```python
from build123d import *

# Parameters (mm, degrees)
ESBO_O1_W                = 2
ESBO_O1_H                = 2
RESSALTO_EXTRUS_O1_DEPTH = 100
RESSALTO_EXTRUS_O2_DEPTH = 2
RESSALTO_EXTRUS_O3_DEPTH = 2
ESBO_O4_R                = 1.75
CORTE_EXTRUS_O1_DEPTH    = 2
ESBO_O5_R                = 1.75
CORTE_EXTRUS_O2_DEPTH    = 2


with BuildPart() as part:
    # Esboço1 → Ressalto-extrusão1 (new body)
    with BuildSketch(Plane(origin=(0, 0, 0), x_dir=(1, 0, 0), z_dir=(0, 1, 0))):
        with Locations((1, 1)):
            Rectangle(ESBO_O1_W, ESBO_O1_H)
    extrude(amount=RESSALTO_EXTRUS_O1_DEPTH)

    # Esboço2 → Ressalto-extrusão2 (add)
    with BuildSketch(Plane.XY):
        Polygon((2, 0), (100, 0), (2, 100), align=None)
    extrude(amount=-RESSALTO_EXTRUS_O2_DEPTH)

    # Esboço3 → Ressalto-extrusão3 (add)
    with BuildSketch(Plane.ZY):
        Polygon((-2, 0), (-2, 100), (-100, 0), align=None)
    extrude(amount=-RESSALTO_EXTRUS_O3_DEPTH)

    # Esboço4 → Corte-extrusão1 (cut)
    with BuildSketch(Plane.ZY):
        with Locations((-10, 15)):
            Circle(ESBO_O4_R)
        with Locations((-10, 30)):
            Circle(ESBO_O4_R)
        with Locations((-10, 85)):
            Circle(ESBO_O4_R)
        with Locations((-10, 70)):
            Circle(ESBO_O4_R)
        with Locations((-55, 15)):
            Circle(ESBO_O4_R)
        with Locations((-70, 15)):
            Circle(ESBO_O4_R)
    extrude(amount=-CORTE_EXTRUS_O1_DEPTH, mode=Mode.SUBTRACT)

    # Esboço5 → Corte-extrusão2 (cut)
    with BuildSketch(Plane.XY):
        with Locations((10, 15)):
            Circle(ESBO_O5_R)
        with Locations((10, 30)):
            Circle(ESBO_O5_R)
        with Locations((10, 85)):
            Circle(ESBO_O5_R)
        with Locations((10, 70)):
            Circle(ESBO_O5_R)
        with Locations((70, 15)):
            Circle(ESBO_O5_R)
        with Locations((55, 15)):
            Circle(ESBO_O5_R)
    extrude(amount=-CORTE_EXTRUS_O2_DEPTH, mode=Mode.SUBTRACT)


solid = part.part
```
Design review of the part built by this model. Coordinates are the model's own, in mm. A direction names the side the tool comes from. Give positions to 0.01 mm unless a question says otherwise; leave off trailing zeros. Order: outer loops, then holes, each group sorted by start corner. A loop starts at its lowest first (then second) coordinate and runs counter-clockwise, first axis right, second up. Notation, with made-up numbers: (-30, 43.5) - (14, 43.5) arc R35 cw to (14, 82.5) - close; hole circle Ø10 at (65.5, 88.25). An arc over 180 degrees is marked (long way). Use a Markdown table: item, result. Add a question column.
(1) Add section D-D on y = 30. Give the boundary of the cut face in (x, z).
(2) Mouldability with a two-part tool opening along Z and no side actions: class faces 3 (the face through (0.986, 15.526, -68.331)), 4 (the face through (0.986, 50.7, -50.314)), 5 (the face through (51.686, 49.3, -0.986)) as +Z half, -Z half, draft (parallel to the pull), parting line (faces both ways), or undercut.
(3) Machinability: for faces 1 (the face through (9.772, 16.735, -0.986)), 2 (the face through (2, 28, -30)), which of the approach directions +Z, -Z, +X, -X, +Y, -Y give a long, thin tool a straight path to every point of the face, cutting with its end or side? Answer none if there is none.
(4) Add section B-B on z = -55. Give the boundary of the cut face in (x, y).
(5) Add section A-A on y = 15. Give the number of separate pieces and of enclosed holes in the cut face, then the cut area to 3 significant figures.
(6) Add section C-C on x = 10. Give the boundary of the cut face in (y, z).
(7) Wall thickness on probe 1 along Y at (x, z) = (1, -10); probe 2 along Z at (x, y) = (50, 21); probe 3 along X at (y, z) = (34.5, -15.5): over which ranges is each line inside the solid? List them lowest first. Write a range as [from, to].
(8) Clearance check with flat-ended pins moving along their axes: P1, Ø3, axis at x = 10, y = 30, coming from the -Z side; P2, Ø5.5, axis at x = 10, y = 15, coming from the -Z side. State where each tip first meets the part, or that it passes through.
Report:
| question | item | result |
|---|---|---|
| 1 | outline | (0, -70.6) - (2, -70.6) - (2, -11.75) - (0, -11.75) - close; (0, -8.25) - (2, -8.25) - (2, -2) - (8.25, -2) - (8.25, 0) - (0, 0) - close; (11.75, -2) - (70.6, -2) - (70.6, 0) - (11.75, 0) - close |
| 2 | face 3 | undercut |
| 2 | face 4 | -Z half |
| 2 | face 5 | draft |
| 3 | face 1 | +Z, -Z |
| 3 | face 2 | -Z, +X, +Y, -Y |
| 4 | outline | (0, 0) - (2, 0) - (2, 13.25) - (0, 13.25) - close; (0, 16.75) - (2, 16.75) - (2, 45.92) - (0, 45.92) - close |
| 5 | separate pieces | 7 |
| 5 | enclosed holes | 0 |
| 5 | area | 295 mm² |
| 6 | outline | (0, -2) - (13.25, -2) - (13.25, 0) - (0, 0) - close; (16.75, -2) - (28.25, -2) - (28.25, 0) - (16.75, 0) - close; (31.75, -2) - (68.25, -2) - (68.25, 0) - (31.75, 0) - close; (71.75, -2) - (83.25, -2) - (83.25, 0) - (71.75, 0) - close; (86.75, -2) - (91.84, -2) - (91.84, 0) - (86.75, 0) - close |
| 7 | probe 1 | y = [0, 13.25], [16.75, 28.25], [31.75, 68.25], [71.75, 83.25], [86.75, 91.84] |
| 7 | probe 2 | z = [-2, 0] |
| 7 | probe 3 | x = [0, 2] |
| 8 | P1 | passes through |
| 8 | P2 | stops at z = -2 |
